Autodesk Inventor part; units mm, degrees
ref_plane "YZ Plane" through (0, 0, 0) normal (1, 0, 0) x (0, 1, 0)
ref_plane "XZ Plane" through (0, 0, 0) normal (0, 1, 0) x (-1, 0, 0)
ref_plane "XY Plane" through (0, 0, 0) normal (0, 0, 1) x (1, 0, 0)
sketch "Sketch1" plane through (0, 0, 0) normal (0, 1, 0) x (-1, 0, 0)
  line L0 (0, 0) -> (44.45, 0)
  line L1 (44.45, 0) -> (44.45, -44.45)
  line L2 (44.45, -44.45) -> (0, -44.45)
  line L3 (0, -44.45) -> (0, 0)
  dimension "d0" = 44.45
  dimension "d1" = 44.45
extrude "Extrusion1" add sketch "Sketch1" along normal blind 3.175
sketch "Sketch2" plane through (-44.45, 0, 0) normal (0, 0, 1) x (1, 0, 0)
  line L0 (0, 50.8) -> (44.45, 50.8)
  line L1 (44.45, 0) -> (0, 0)
  line L2 (22.225, 50.8) -> (22.225, 54.352)
  line L3 (22.225, 0) -> (22.225, -5.76)
  line L4 (0, 50.8) -> (0.0188, 3.175)
  line L5 (0.0188, 3.175) -> (44.4312, 3.175)
  line L6 (44.4312, 3.175) -> (44.45, 50.8)
  line L7 (0, 3.175) -> (44.45, 3.175)
  dimension "d4" = 44.45
  dimension "d5" = 50.8
  dimension "d6" = 0
  dimension "d9" = 0
extrude "Extrusion2" add sketch "Sketch2" against normal blind 3.175
properties part number "Bottom Elevator Bracket Square"
Input: part model. Units: mm. Frame: model coordinates. A direction names the side the tool comes from. Coordinates: 2 decimals unless noted, no trailing zeros. Loops run counter-clockwise (first coordinate to the right, second up) from the corner with the lowest first, then second, coordinate; pieces in that order, holes last.
Q1. Set-up query: faces 1 (the flat face through (0, 2, -23)), 2 (the flat face through (-23, 27, -3.175)). Return all of +Z, -Z, +X, -X, +Y, -Y with unobstructed straight access to the full face (end or side cutting, diameter ignored); none if empty.
Results are:
face 1: +Z, -Z, +X, +Y, -Y
face 2: -Z, +X, -X, +Y
Q2. Line query: line 1 along Y through (x, z) = (-28.5, -9.5) (3 decimals); line 2 along Z through (x, y) = (-25, 13) (3 decimals). Output: solid intervals per line, ascending.
Results are:
line 1: y = 0 to 3.175
line 2: z = -3.175 to 0
Q3. Section C-C, the plane y = 35. Return the cut outline in (x, z) (3 decimals).
Results are:
outline: (-44.444, -3.175) - (-0.006, -3.175) - (-0.006, 0) - (-44.444, 0) - close
Q4. Section A-A, the plane x = -15.5. Return the cut outline in (y, z) (3 decimals).
Results are:
outline: (0, -44.45) - (3.175, -44.45) - (3.175, -3.175) - (50.8, -3.175) - (50.8, 0) - (0, 0) - close
Q5. Section B-B, the plane z = -41. Return the cut outline in (x, y) (3 decimals), and give its area (3 significant figures).
Results are:
outline: (-44.45, 0) - (0, 0) - (0, 3.175) - (-44.45, 3.175) - close
area: 141 mm2
Q6. Contact query for flat-ended pins moving along their axis: pin 1 (8 mm diameter, centred on x = -28.5, z = -16.5, fed in from +Y) (3 decimals); pin 2 (1.6 mm diameter, centred on y = 29, z = -2, fed in from +X). Output: stop coordinate, or through.
Results are:
pin 1: stops at y = 3.175
pin 2: stops at x = -0.01
